Design review of the part built by this model. Coordinates are the model's own, in mm. A direction names the side the tool comes from. Coordinates: 2 decimals unless noted, no trailing zeros. Write each loop counter-clockwise with the first axis right and the second up, starting at its lowest first coordinate (ties: lowest second). Pieces come first, ordered by that corner, then holes. Notation, with made-up numbers: (68.25, 87) - (108.25, 87) arc R17 ccw to (108.25, 93) - close; hole circle Ø2 at (-13.75, 46.5). An arc over 180 degrees is marked (long way). Answer as a JSON object with one key per item and string values.
```python
from build123d import *

# Parameters (mm, degrees)
F0_R     = 28.5
F1_DEPTH = 3
F2_R     = 26
F2_R_2   = 24
F3_DEPTH = 1
F4_R     = 12.5
F5_DEPTH = 7
F6_R     = 4
F7_DEPTH = 3


with BuildPart() as f1:
    # F0 (on Top) → F1 (new body)
    with BuildSketch(Plane.XY):
        Circle(F0_R)
    extrude(amount=F1_DEPTH)

    # F2 (on face) → F3 (cut)
    with BuildSketch(Plane.XY.offset(3)):
        Circle(F2_R)
        Circle(F2_R_2, mode=Mode.SUBTRACT)
    extrude(amount=-F3_DEPTH, mode=Mode.SUBTRACT)

    # F4 (on face) → F5 (join)
    with BuildSketch(Plane.XY.offset(3)):
        Circle(F4_R)
    extrude(amount=F5_DEPTH)

    # F6 (on face) → F7 (cut)
    with BuildSketch(Plane.XY.offset(3)):
        with Locations((0, 18.25)):
            Circle(F6_R)
    extrude(amount=-F7_DEPTH, mode=Mode.SUBTRACT)


solid = f1.part
```
(1) Tool access review of faces 1 (the face through (-23.977, 1.055, 2.507)), 2 (the face through (0, 0, 10)): name each direction out of +Z, -Z, +X, -X, +Y, -Y from which nothing blocks a thin tool from reaching the whole face with its end or side.
Solved:
{"face 1": "+Z", "face 2": "+Z, +X, -X, +Y, -Y"}
(2) Take a section at A-A, the plane x = 0. Write out the cut boundary in (y, z).
Solved:
{"outline": "(-28.5, 0) - (14.25, 0) - (14.25, 3) - (12.5, 3) - (12.5, 10) - (-12.5, 10) - (-12.5, 3) - (-24, 3) - (-24, 2) - (-26, 2) - (-26, 3) - (-28.5, 3) - close; (22.25, 0) - (28.5, 0) - (28.5, 3) - (26, 3) - (26, 2) - (24, 2) - (24, 3) - (22.25, 3) - close"}
(3) Take a section at C-C, the plane y = 0. Write out the cut boundary in (x, z).
Solved:
{"outline": "(-28.5, 0) - (28.5, 0) - (28.5, 3) - (26, 3) - (26, 2) - (24, 2) - (24, 3) - (12.5, 3) - (12.5, 10) - (-12.5, 10) - (-12.5, 3) - (-24, 3) - (-24, 2) - (-26, 2) - (-26, 3) - (-28.5, 3) - close"}
(4) The part is to be moulded in two halves that separate along Y. For faces 3 (the face through (23, -13, 3)), 4 (the face through (26.327, -10.916, 1.479)), 5 (the face through (-0.521, 22.216, 1.521)), say which applies: pulls with the +Y half, pulls with the -Y half, needs draft (parallel to the pull), parting line crosses it, or undercut.
Solved:
{"face 3": "needs draft", "face 4": "parting line crosses it", "face 5": "undercut"}
(5) Take a section at B-B, the plane y = 16.5. Write out the cut boundary in (x, z), and give its area (3 significant figures).
Solved:
{"outline": "(-23.24, 0) - (-3.6, 0) - (-3.6, 3) - (-17.43, 3) - (-17.43, 2) - (-20.09, 2) - (-20.09, 3) - (-23.24, 3) - close; (3.6, 0) - (23.24, 0) - (23.24, 3) - (20.09, 3) - (20.09, 2) - (17.43, 2) - (17.43, 3) - (3.6, 3) - close", "area": "113 mm^2"}
(6) Take a section at D-D, the plane z = 8.5. Write out the cut boundary in (x, y), and give its area (3 significant figures).
Solved:
{"outline": "circle Ø25 at (0, 0)", "area": "491 mm^2"}
(7) For pin 1 (1 mm diameter, centred on x = 0, y = -18.5, fed in from +Z); pin 2 (3 mm diameter, centred on x = 2, z = 6.5, fed in from +Y); pin 3 (3 mm diameter, centred on y = 17.5, z = 2, fed in from +X), all flat-tipped, find the tip position at first contact; note any pin that passes through.
Solved:
{"pin 1": "stops at z = 3", "pin 2": "stops at y = 12.49", "pin 3": "stops at x = 23.58"}
(8) To check wall thickness, follow line 1 (Y direction, x = 15.5, z = 2.5); line 2 (X direction, y = -15, z = 2.5) (3 decimals); line 3 (Z direction, x = -13, y = -11). State the ranges of each line that lie inside material, in increasing order. Write a range as from..to.
Solved:
{"line 1": "y = -23.92..-20.87, -18.32..18.32, 20.87..23.92", "line 2": "x = -24.233..-21.237, -18.735..18.735, 21.237..24.233", "line 3": "z = 0..3"}
